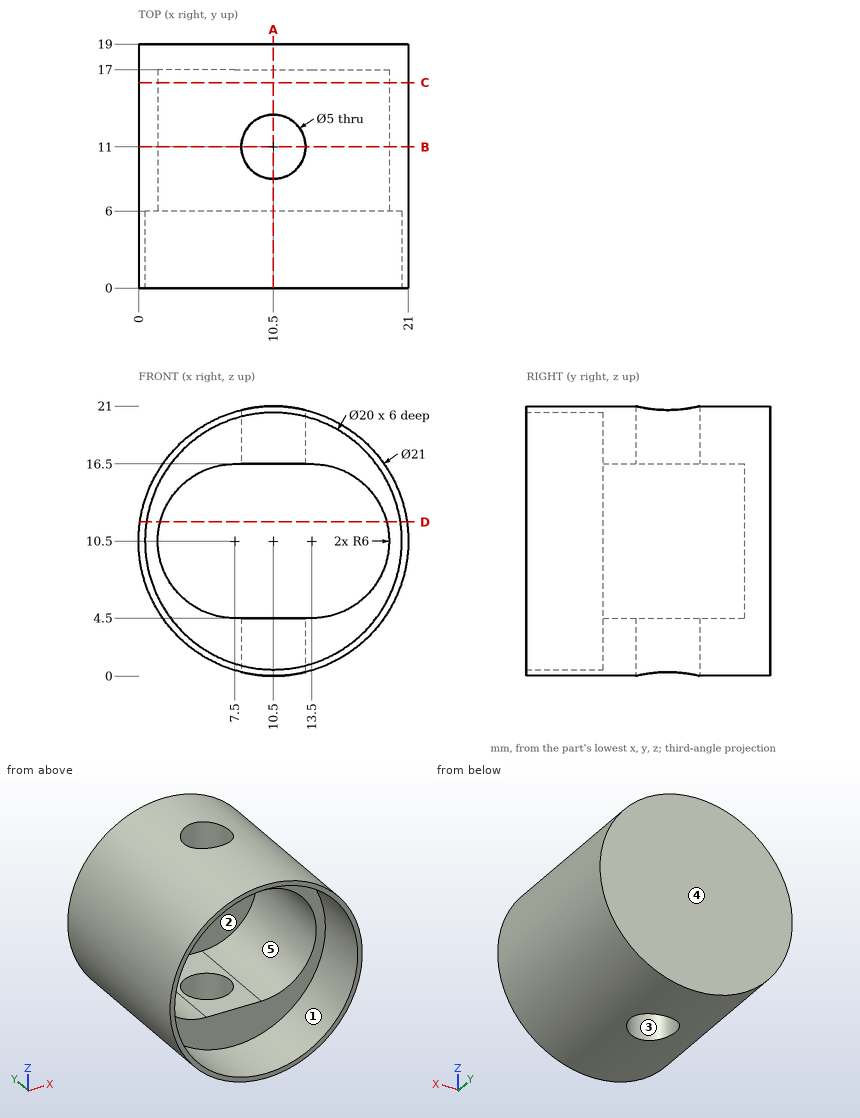
Drawing for the job (mm, zero at the part's lowest x, y, z). A direction names the side the tool comes from. Give positions to 0.01 mm unless a question says otherwise; leave off trailing zeros. Loops run counter-clockwise (first coordinate to the right, second up) from the corner with the lowest first, then second, coordinate; pieces in that order, holes last. Notation, with made-up numbers: (63, 48.25) - (86, 48.25) arc R17 cw to (86, 62.25) - close; hole circle Ø5 at (72, -25.75). An arc over 180 degrees is marked (long way). Write item = value, one per line. Start each with the question number.
1) Tool access for the marked faces 4 and 5: list every direction of +Z, -Z, +X, -X, +Y, -Y with a clear straight run to the whole face (end or side of a thin tool).
2) Probe probe 1 along X at (y, z) = (4, 10.5); probe 2 along Z at (x, y) = (9.75, 4); probe 3 along Y at (x, z) = (8.75, 10.5). List the from-to ranges inside material, lowest first. Write a range as from..to.
3) Band-saw the part on D-D on z = 12. Give the cut face in (x, y).
4) Drop flat-ended pins along their axis: pin 1 Ø5 at (y, z) = (9.5, 3.5) entering from +X; pin 2 Ø3 at (x, y) = (10.5, 11) entering from -Z; pin 3 Ø3 at (x, y) = (17, 10.5) entering from -Z; pin 4 Ø5 at (y, z) = (9, 14.5) entering from -X. Give the stop position or say it passes through.
5) Band-saw the part on A-A on x = 10.5. Give the cut face in (y, z), plus the area to 3 significant figures.
6) Band-saw the part on C-C on y = 16. Give the cut face in (x, z), plus the area to 3 significant figures.
7) Band-saw the part on B-B on y = 11. Give the cut face in (x, z), plus the area to 3 significant figures.
8) Pull direction Y, two halves, no side cores. Call the marked faces 1, 2 and 3: +Y half, -Y half, draft (parallel to the pull), parting line (faces both ways), or undercut.
Final values:
q1.face_4 = +Z, -Z, +X, -X, +Y
q1.face_5 = -Y
q2.probe_1 = 0..0.5, 20.5..21
q2.probe_2 = 0.03..0.53, 20.47..20.97
q2.probe_3 = 17..19
q3.outline = (0.11, 0) - (0.61, 0) - (0.61, 6) - (1.69, 6) - (1.69, 17) - (19.31, 17) - (19.31, 6) - (20.39, 6) - (20.39, 0) - (20.89, 0) - (20.89, 19) - (0.11, 19) - close
q4.pin_1 = 19.99
q4.pin_2 = through
q4.pin_3 = 1.27
q4.pin_4 = 0.11
q5.outline = (0, 0) - (8.5, 0) - (8.5, 4.5) - (6, 4.5) - (6, 0.5) - (0, 0.5) - close; (0, 20.5) - (6, 20.5) - (6, 16.5) - (8.5, 16.5) - (8.5, 21) - (0, 21) - close; (13.5, 0) - (19, 0) - (19, 21) - (13.5, 21) - (13.5, 16.5) - (17, 16.5) - (17, 4.5) - (13.5, 4.5) - close
q5.area = 102 mm²
q6.outline = circle Ø21 at (10.5, 10.5); hole (7.5, 4.5) - (13.5, 4.5) arc R6 ccw to (13.5, 16.5) - (7.5, 16.5) arc R6 ccw to start
q6.area = 161 mm²
q7.outline = (7.5, 4.5) arc R6 cw to (7.5, 16.5) - (8, 16.5) - (8, 20.7) arc R10.5 ccw to (8, 0.3) - (8, 4.5) - close; (13, 0.3) arc R10.5 ccw to (13, 20.7) - (13, 16.5) - (13.5, 16.5) arc R6 cw to (13.5, 4.5) - (13, 4.5) - close
q7.area = 117 mm²
q8.face_1 = draft
q8.face_2 = -Y half
q8.face_3 = undercut
